Autodesk Inventor part; units mm, degrees
ref_plane "YZ Plane" through (0, 0, 0) normal (1, 0, 0) x (0, 1, 0)
ref_plane "XZ Plane" through (0, 0, 0) normal (0, 1, 0) x (-1, 0, 0)
ref_plane "XY Plane" through (0, 0, 0) normal (0, 0, 1) x (1, 0, 0)
sketch "Skizze1" plane through (0, 0, 0) normal (0, 1, 0) x (-1, 0, 0)
  line L0 (8.5, -4) -> (-8.5, -4)
  line L1 (-8.5, -4) -> (-8.5, 3)
  line L2 (-8.5, 3) -> (8.5, 3)
  line L3 (8.5, 3) -> (8.5, -4)
  line L4 (-11.9, 0) -> (11.9, 0) construction
  line L5 (0, -5.4) -> (0, 4.4) construction
  point P0 (0, 0)
  dimension "d0" = 17
  dimension "d1" = 7
  dimension "d60" = 3
extrude "Extrusion1" add sketch "Skizze1" along normal blind 4.4
sketch "Skizze2" plane through (0, 0, 0) normal (0, -1, 0) x (1, 0, 0)
  line L0 (-11.9, 0) -> (11.9, 0)
  line L1 (0, 4.4) -> (0, -5.4)
  point P0 (0, 0)
  point P1 (-6, 0.8)
  point P2 (6, 0.8)
  dimension "d5" = 0.8
  dimension "d6" = 6
hole "Bohrung1" at (-6, 0, 0.8) at (6, 0, 0.8) direction (0, 1, 0) diameter 1.9 end through all
sketch "Skizze5" plane through (0, 0, 0) normal (0, -1, 0) x (1, 0, 0)
  line L0 (8.5, -4) -> (-8.5, -4)
  line L1 (8.5, 3) -> (8.5, -4)
  line L2 (-8.5, -4) -> (8.5, -4)
  line L3 (8.5, -4) -> (8.5, -3)
  line L4 (8.5, -3) -> (-8.5, -3)
  line L5 (-8.5, -3) -> (-8.5, -4)
  point P0 (0, 0)
  dimension "d29" = 1
extrude "Extrusion4" [suppressed]
sketch "Skizze6" plane through (0, 0, 0) normal (0, -1, 0) x (1, 0, 0)
  line L0 (8.5, -4) -> (8.5, 3)
  line L1 (8.5, 3) -> (-8.5, 3)
  line L2 (-8.5, 3) -> (-8.5, -4)
  circle A0 centre (-6, 0.8) radius 0.95
  circle A1 centre (6, 0.8) radius 0.95
  line L3 (8.5, 3) -> (-8.5, 3)
  line L4 (-3, 3) -> (3, 3)
  line L5 (3, 3) -> (3, -2)
  line L6 (3, -2) -> (-3, -2)
  line L7 (-3, -2) -> (-3, 3)
  line L8 (0, 4.4) -> (0, -5.4)
  line L9 (-8.5, -4) -> (8.5, -4)
  point P0 (0, 0)
  point P1 (0, 3)
  dimension "d32" = 6
  dimension "d58" = 2
  dimension "d59" = 2
extrude "Extrusion5" cut sketch "Skizze6" against normal through all contours L5 L6 L8 L1 | L6 L7 L1 L8
sketch "Skizze7" plane through (-8.5, -0.4, -2) normal (0, 0, 1) x (1, 0, 0)
  line L0 (0, 0) -> (1, 0)
  line L1 (1, 0) -> (1, 0.4)
  line L2 (1, 0.4) -> (0, 0.4)
  line L3 (0, 0.4) -> (0, 0)
  line L4 (17, 0) -> (0, 0)
  line L5 (11.5, 0.4) -> (17, 0.4)
  line L6 (17, 0) -> (16, 0)
  line L7 (16, 0) -> (16, 0.4)
  line L8 (16, 0.4) -> (17, 0.4)
  line L9 (17, 0.4) -> (17, 0)
  point P0 (8.5, 0.4)
  dimension "d35" = 1
  dimension "d36" = 1
extrude "Extrusion6" [suppressed]
chamfer "Fase4" [suppressed]
chamfer "Fase6" distance 1.5 distance2 4 1 edges at (-3, 0, 0.5) measured on face at (1, 0, -3.3333)
chamfer "Fase7" distance 1.5 distance2 4 1 edges at (3, 0, 0.5) measured on face at (1, 0, -3.3333)
fillet "Rundung3" radius 2 4 edges at (-3.75, 2, 3) (-3, 4.2, 3) (3.75, 2, 3) (3, 4.2, 3)
sketch "Skizze8" plane through (0, 0, 0) normal (0, -1, 0) x (1, 0, 0)
  line L0 (-3, 3) -> (-7.5, 3)
  line L1 (-7.5, 3) -> (-7.5, -2)
  line L2 (-7.5, -2) -> (-3, -2)
  line L3 (-3, -2) -> (-3, 3)
  circle A0 centre (-6, 1) radius 0.95
  line L4 (3, 3) -> (3, -2)
  line L5 (3, -2) -> (7.5, -2)
  line L6 (7.5, -2) -> (7.5, 3)
  line L7 (7.5, 3) -> (3, 3)
  circle A1 centre (6, 1) radius 0.95
  line L8 (-7.5, 3) -> (-7.5, -2)
  line L9 (-7.5, -2) -> (-3, -2)
  line L10 (-3, -2) -> (-3, 3)
  line L11 (-3, 3) -> (-7.5, 3)
  line L12 (7.5, -2) -> (7.5, 3)
  line L13 (3, 3) -> (3, -2)
  line L14 (3, -2) -> (7.5, -2)
  line L15 (7.5, 3) -> (3, 3)
properties part number "LED Schirm"
Model file for the job. Use its own axes, mm. A direction names the side the tool comes from. Coordinates: 2 decimals unless noted, no trailing zeros. Loops run counter-clockwise (first coordinate to the right, second up) from the corner with the lowest first, then second, coordinate; pieces in that order, holes last. Notation, with made-up numbers: (-10.75, 8.25) - (-4.75, 8.25) arc R25 ccw to (-4.75, 32.25) - close; hole circle Ø9 at (81, -6). An arc over 180 degrees is marked (long way). Write item = value, one per line. Start each with the question number.
Item 1: 3-axis set-ups, long thin cutter, end or side, ignore diameter. For faces 1 (the face through (4.4, 1.9, 2.4)), 2 (the face through (-3.374, 4.247, 2.165)), 3 (the face through (-6.8, 2.23, 0.29)): which of +Z, -Z, +X, -X, +Y, -Y reach the whole face in a straight line?
Item 2: Saw through at B-B, the plane z = -1.75. List the corners of the cut face in (x, y).
Item 3: Pull direction X, two halves, no side cores. Call faces 4 (the face through (-8.5, 2, 0)), 5 (the face through (-7, 2, 3)), 6 (the face through (-3.74, 2.03, -0.52)): +X half, -X half, draft (parallel to the pull), parting line (faces both ways), or undercut.
Item 4: Saw through at A-A, the plane z = 0.8. List the corners of the cut face in (x, y), then the cut area to 3 significant figures.
Item 5: Wall check: probe 1 along X at (y, z) = (0.95, 1.25); probe 2 along X at (y, z) = (2.95, 0.8); probe 3 along Z at (x, y) = (6, 1.35). Give the ranges that are in metal, low to high. Write a range as [from, to].
Item 6: Saw through at C-C, the plane y = 1.45. State how many separate pieces and enclosed holes the cut face has, then the cut area to 3 significant figures.
Item 7: Drop a flat-ended pin along its axis: pin 1 Ø1 at (x, y) = (1, 2.5) entering from +Z. Give the stop position or say it passes through.
Item 8: Saw through at D-D, the plane x = -2. List the corners of the cut face in (y, z).
Answers:
q1.face_1 = +Z, -Y
q1.face_2 = +Z, +Y, -Y
q1.face_3 = +Y, -Y
q2.outline = (-8.5, 0) - (-4.5, 0) - (-3, 4) - (-3, 4.4) - (-8.5, 4.4) - close; (3, 4) - (4.5, 0) - (8.5, 0) - (8.5, 4.4) - (3, 4.4) - close
q3.face_4 = -X half
q3.face_5 = draft
q3.face_6 = undercut
q4.outline = (-8.5, 0) - (-6.95, 0) - (-6.95, 4.4) - (-8.5, 4.4) - close; (-5.05, 0) - (-4.5, 0) - (-3, 4) - (-3, 4.4) - (-5.05, 4.4) - close; (3, 4) - (4.5, 0) - (5.05, 0) - (5.05, 4.4) - (3, 4.4) - close; (6.95, 0) - (8.5, 0) - (8.5, 4.4) - (6.95, 4.4) - close
q4.area = 25.7 mm2
q5.probe_1 = [-8.5, -6.84], [-5.16, -4.16], [4.16, 5.16], [6.84, 8.5]
q5.probe_2 = [-8.5, -6.95], [-5.05, -3.39], [3.39, 5.05], [6.95, 8.5]
q5.probe_3 = [-4, -0.15], [1.75, 3]
q6.separate_pieces = 1
q6.enclosed_holes = 2
q6.area = 71.9 mm2
q7.pin_1 = -2
q8.outline = (0, -4) - (4.4, -4) - (4.4, -2) - (0, -2) - close
